Source: CAD feature listing. Evaluate the final solid. Frame: model axes, mm. A direction names the side the tool comes from. Give positions to 0.01 mm unless a question says otherwise; leave off trailing zeros. Order: outer loops, then holes, each group sorted by start corner. A loop starts at its lowest first (then second) coordinate and runs counter-clockwise, first axis right, second up. Notation, with made-up numbers: (50.25, 50.5) - (77.25, 50.5) arc R12 cw to (77.25, 66.5) - close; hole circle Ø4 at (-13.5, 50). An arc over 180 degrees is marked (long way). Answer as CSV lines item,"result".
```python
from build123d import *

# Parameters (mm, degrees)
F0_R     = 4
F1_DEPTH = 15
F2_R     = 1.533854
F3_DEPTH = 25


with BuildPart() as f1:
    # F0 (on Right) → F1 (new body, symmetric)
    with BuildSketch(Plane.YZ):
        Polygon((5.351402, 22), (-5.351402, 22), (-11.303023, 16.958306), (-17, 16.958306), (-17, 0), (-6, 0), (-6, 1.75), (6, 1.75), (6, 0), (17, 0), (17, 16.958306), (11.303023, 16.958306), align=None)
        with Locations((0, 11.875)):
            Circle(F0_R, mode=Mode.SUBTRACT)
    extrude(amount=F1_DEPTH, both=True)

    # F2 (on Top) → F3 (cut)
    with BuildSketch(Plane.XY):
        with Locations((-8.75, -12.5)):
            Circle(F2_R)
        with Locations((-8.75, 12.5)):
            Circle(F2_R)
        with Locations((8.75, 12.5)):
            Circle(F2_R)
        with Locations((8.75, -12.5)):
            Circle(F2_R)
    extrude(amount=F3_DEPTH, mode=Mode.SUBTRACT)


solid = f1.part
```
(1) Cut plane A-A (y = 12.5). Return loops of the section in (x, z), then the cut area to 3 significant figures.
Completed:
outline,"(-15, 0) - (-10.28, 0) - (-10.28, 16.96) - (-15, 16.96) - close; (-7.22, 0) - (7.22, 0) - (7.22, 16.96) - (-7.22, 16.96) - close; (10.28, 0) - (15, 0) - (15, 16.96) - (10.28, 16.96) - close"
area,"405 mm²"
(2) Ray query, line 1 (X direction, y = -12.5, z = 3.75); line 2 (Y direction, x = -8.75, z = 4.5); line 3 (Y direction, x = -8.75, z = 9.25). Return the intervals inside material, ascending. Write a range as from..to.
Completed:
line 1,"-15..-10.28, -7.22..7.22, 10.28..15"
line 2,"-17..-14.03, -10.97..10.97, 14.03..17"
line 3,"-17..-14.03, -10.97..-3.02, 3.02..10.97, 14.03..17"
(3) Access query for faces 4 (the flat face through (0, -14, 16.958)), 5 (the flat face through (0, 14, 16.958)), 6 (the flat face through (0, 0, 22)), 7 (the flat face through (0, 6, 1)). Directions: +Z, -Z, +X, -X, +Y, -Y. A direction counts if a zero-diameter tool reaches every point of the face in a straight line with its end or side. Return the directions, or none.
Completed:
face 4,"+Z, +X, -X, -Y"
face 5,"+Z, +X, -X, +Y"
face 6,"+Z, +X, -X, +Y, -Y"
face 7,"-Z, +X, -X"
(4) Mould query, pull axis X, two halves, no side actions, for faces 1 (the flat face through (15, 0, 6)), 2 (the flat face through (0, 17, 8)), 3 (the cylindrical face through (-8.04, 11.14, 8.52)). Classes: released by +X, released by -X, zero draft, split by the parting line, or undercut.
Completed:
face 1,"released by +X"
face 2,"zero draft"
face 3,"undercut"
(5) Contact query for flat-ended pins moving along their axis: pin 1 (6.5 mm diameter, centred on x = -6, y = -13.5, fed in from +Z); pin 2 (6.5 mm diameter, centred on x = -0.5, y = 14, fed in from +Z). Output: stop coordinate, or through.
Completed:
pin 1,"z = 17.85"
pin 2,"z = 17.43"
(6) Cut plane C-C (x = 8.75). Return loops of the section in (y, z) (3 decimals), then the cut area to 3 significant figures.
Completed:
outline,"(-17, 0) - (-14.034, 0) - (-14.034, 16.958) - (-17, 16.958) - close; (-10.966, 0) - (-6, 0) - (-6, 1.75) - (6, 1.75) - (6, 0) - (10.966, 0) - (10.966, 17.244) - (5.351, 22) - (-5.351, 22) - (-10.966, 17.244) - close; (14.034, 0) - (17, 0) - (17, 16.958) - (14.034, 16.958) - close; hole circle Ø8 at (0, 11.875)"
area,"485 mm²"
(7) Cut plane B-B (z = 5.5). Return loops of the section in (x, y).
Completed:
outline,"(-15, -17) - (15, -17) - (15, 17) - (-15, 17) - close; hole circle Ø3.07 at (-8.75, -12.5); hole circle Ø3.07 at (-8.75, 12.5); hole circle Ø3.07 at (8.75, -12.5); hole circle Ø3.07 at (8.75, 12.5)"
(8) Cut plane D-D (y = 0). Return loops of the section in (x, z) (3 decimals), then the cut area to 4 significant figures.
Completed:
outline,"(-15, 1.75) - (15, 1.75) - (15, 7.875) - (-15, 7.875) - close; (-15, 15.875) - (15, 15.875) - (15, 22) - (-15, 22) - close"
area,"367.5 mm²"
